Could you check a few things on this model? Use its own coordinates, in mm. Face numbers are marked on the shaded views. A direction names the side the tool comes from. Round coordinates to 2 decimals unless told otherwise and drop trailing zeros. Loops run counter-clockwise (first coordinate to the right, second up) from the corner with the lowest first, then second, coordinate; pieces in that order, holes last. Notation, with made-up numbers: (-36.75, 7.25) -> (-3.75, 7.25) arc R14 ccw to (-3.75, 28.25) -> close; hole circle Ø8 at (19.25, 9). An arc over 180 degrees is marked (long way). One line per item, written item: value.
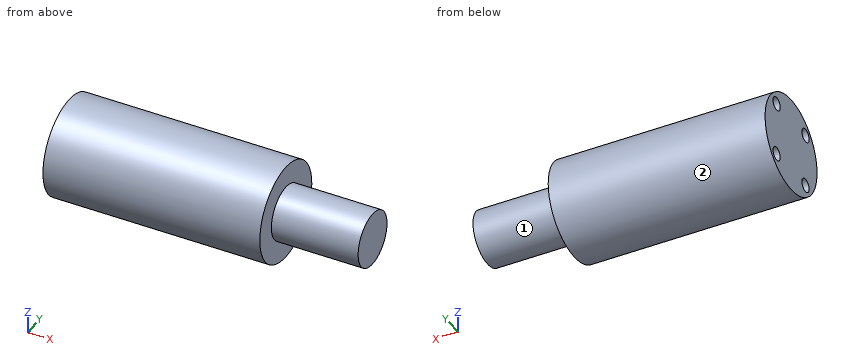
from build123d import *

# Parameters (mm, degrees)
HOLE_WIZARD_M3_1_D     = 2.5
HOLE_WIZARD_M3_1_DEPTH = 5
HOLE_WIZARD_M3_1_TIP   = 0.751075774


with BuildPart() as part:
    # 草图2 → 旋转1 (revolve)
    with BuildSketch(Plane.XY):
        Polygon((0, 0), (0, 9), (40, 9), (40, 5), (56, 5), (56, 0), align=None)
    revolve(axis=Axis((56, 0, 0), (-1, 0, 0)))

    # M3 螺纹孔1
    with Locations(Plane.ZY):
        with Locations((-5, 5), (5, 5), (5, -5), (-5, -5)):
            Hole(HOLE_WIZARD_M3_1_D / 2, depth=HOLE_WIZARD_M3_1_DEPTH)
            with Locations((0, 0, -(HOLE_WIZARD_M3_1_DEPTH + HOLE_WIZARD_M3_1_TIP / 2))):  # 118° drill point
                Cone(0, HOLE_WIZARD_M3_1_D / 2, HOLE_WIZARD_M3_1_TIP, mode=Mode.SUBTRACT)


solid = part.part
(1) I'm going to push flat-ended pins straight in: pin 1 Ø5 at (x, z) = (44, -4.5) entering from -Y; pin 2 Ø2 at (x, y) = (48, 2.5) entering from +Z; pin 3 Ø3 at (x, y) = (37.5, -5.5) entering from -Z. Where does each tip first touch, or does it pass through?
Recorded:
pin 1: y = -4.58
pin 2: z = 4.77
pin 3: z = -8.06
(2) If we section it at C-C, the plane x = 31.5: Please give me the cut outline in (y, z).
Recorded:
outline: circle Ø18 at (0, 0)
(3) If we section it at A-A, the plane z = 0: Please give me the cut outline in (x, y), then the cut area to 3 significant figures.
Recorded:
outline: (0, -9) -> (40, -9) -> (40, -5) -> (56, -5) -> (56, 5) -> (40, 5) -> (40, 9) -> (0, 9) -> close
area: 880 mm²
(4) For the marked faces 1 and 2, which set-ups out of +Z, -Z, +X, -X, +Y, -Y let a thin tool reach every point of the face, with its end or its side?
Recorded:
face 1: +X
face 2: +X, -X
(5) If I drill on L1, parallel to Z at x = 3.8, y = 5; L2, parallel to X at y = 0.25, z = 8, over which ranges is the centre line in solid material (lowest first)?
Recorded:
L1: -7.48 to -6.25, -3.75 to 3.75, 6.25 to 7.48
L2: 0 to 40
(6) If we section it at D-D, the plane z = 7: Please give me the cut outline in (x, y), then the cut area to 3 significant figures.
Recorded:
outline: (0, -5.66) -> (40, -5.66) -> (40, 5.66) -> (0, 5.66) -> close
area: 453 mm²
